Design review of the part built by this model. Coordinates are the model's own, in mm. Face numbers are marked on the shaded views. A direction names the side the tool comes from. Round coordinates to 2 decimals unless told otherwise and drop trailing zeros. Loops run counter-clockwise (first coordinate to the right, second up) from the corner with the lowest first, then second, coordinate; pieces in that order, holes last. Notation, with made-up numbers: M -9,45.25 L 24,45.25 A13 cw 24,70.25 Z; hole C -4.75,15.25 d11. An arc over 180 degrees is marked long. Use a Markdown table: item, result.
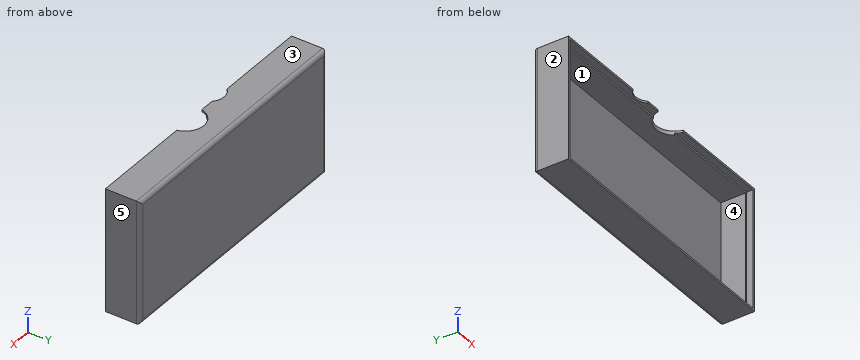
Autodesk Inventor part; units mm, degrees
sketch "Sketch8" plane through (0, 0, 0) normal (0, 1, 0) x (-1, 0, 0)
  line L0 (101.5, -46.5) -> (-101.5, -46.5)
  line L1 (-101.5, -46.5) -> (-101.5, 46.5)
  line L2 (-101.5, 46.5) -> (101.5, 46.5)
  line L3 (101.5, 46.5) -> (101.5, -46.5)
  line L4 (101.5, -46.5) -> (-101.5, 46.5) construction
  line L5 (-101.5, -46.5) -> (101.5, 46.5) construction
  point P0 (0, 0)
  dimension "d19" = 203
  dimension "d20" = 93
extrude "Extrusion4" add sketch "Sketch8" along normal blind 26.5
shell "Shell3" thickness 3 removed faces 1 at (-33.8333, 0, 15.5)
sketch "Sketch11" plane through (0, 0, 0) normal (0, 1, 0) x (-1, 0, 0)
  line L0 (-100, 45) -> (100, 45)
  line L1 (100, 45) -> (100, -45)
  line L2 (100, -45) -> (-100, -45)
  line L3 (-100, -45) -> (-100, 45)
  line L4 (-100, 45) -> (100, -45) construction
  line L5 (100, 45) -> (-100, -45) construction
  point P0 (0, 0)
  dimension "d28" = 200
  dimension "d29" = 90
extrude "Extrusion6" cut sketch "Sketch11" along normal blind 5
fillet "Fillet1" radius 3 4 edges at (0, 26.5, 46.5) (101.5, 26.5, 0) (0, 26.5, -46.5) (-101.5, 26.5, 0)
sketch "Sketch13" plane through (-101.5, 0, 46.5) normal (0, 0, 1) x (1, 0, 0)
  circle A0 centre (111.5, -3) radius 14
  circle A1 centre (78.5, -8) radius 11.5
  line L0 (-40.6, 0) -> (243.6, 0)
  line L1 (203, 0) -> (203, 23.5)
  point P0 (101.5, 0)
  dimension "d74" = 28
  dimension "d75" = 23
  dimension "d76" = 3
  dimension "d77" = 91.5
  dimension "d78" = 124.5
  dimension "d79" = 8
extrude "Extrusion8" cut sketch "Sketch13" against normal blind 10
properties part number "top"
1. Take a section at D-D on x = 4. Give the boundary of the cut face in (y, z), and give its area (3 significant figures).
Check values:
| item | result |
|---|---|
| outline | M 0,-46.5 L 23.5,-46.5 A3 ccw 26.5,-43.5 L 26.5,43.5 A3 ccw 23.5,46.5 L 9.65,46.5 L 9.65,43.5 L 23.5,43.5 L 23.5,-43.5 L 5,-43.5 L 5,-45 L 0,-45 Z |
| area | 380 mm² |
2. Take a section at B-B on x = 83.5. Give the boundary of the cut face in (y, z), and give its area (3 significant figures).
Check values:
| item | result |
|---|---|
| outline | M 0,-46.5 L 23.5,-46.5 A3 ccw 26.5,-43.5 L 26.5,43.5 A3 ccw 23.5,46.5 L 0,46.5 L 0,45 L 5,45 L 5,43.5 L 23.5,43.5 L 23.5,-43.5 L 5,-43.5 L 5,-45 L 0,-45 Z |
| area | 401 mm² |
3. Machinability: for the marked faces 1 and 2, which of the approach directions +Z, -Z, +X, -X, +Y, -Y give a long, thin tool a straight path to every point of the face, cutting with its end or side? Answer none if there is none.
Check values:
| item | result |
|---|---|
| face 1 | -Y |
| face 2 | +Z, -Z, -X, +Y, -Y |
4. Insertion check: pin 1 (1 mm diameter, centred on x = 9, y = 7, fed in from +Z); pin 2 (1 mm diameter, centred on x = -51, z = 36, fed in from -Y). Each pin has a flat end and moves straight along its axis. Give the tip position at first contact, or say it passes through.
Check values:
| item | result |
|---|---|
| pin 1 | stops at z = -43.5 |
| pin 2 | stops at y = 23.5 |
5. Wall thickness on line 1 along Z through (x, y) = (-86.5, 17.5); line 2 along X through (y, z) = (11.5, -4.5); line 3 along Z through (x, y) = (-22.5, 3.75): over which ranges is each line inside the solid? List them lowest first. Write a range as from..to.
Check values:
| item | result |
|---|---|
| line 1 | z = -46.5..-43.5, 43.5..46.5 |
| line 2 | x = -101.5..-98.5, 98.5..101.5 |
| line 3 | z = -46.5..-45, 45..46.5 |
6. The part is to be moulded in two halves that separate along X. For the marked faces 3, 4 and 5, say which applies: pulls with the +X half, pulls with the -X half, needs draft (parallel to the pull), parting line crosses it, or undercut.
Check values:
| item | result |
|---|---|
| face 3 | needs draft |
| face 4 | undercut |
| face 5 | pulls with the +X half |
7. Take a section at C-C on z = 17.5. Give the boundary of the cut face in (x, y).
Check values:
| item | result |
|---|---|
| outline | M -101.5,0 L -100,0 L -100,5 L -98.5,5 L -98.5,23.5 L 98.5,23.5 L 98.5,5 L 100,5 L 100,0 L 101.5,0 L 101.5,23.5 A3 ccw 98.5,26.5 L -98.5,26.5 A3 ccw -101.5,23.5 Z |
8. Take a section at A-A on y = 17.5. Give the boundary of the cut face in (x, z).
Check values:
| item | result |
|---|---|
| outline | M -101.5,-46.5 L 101.5,-46.5 L 101.5,46.5 L -101.5,46.5 Z; hole M -98.5,-43.5 L 98.5,-43.5 L 98.5,43.5 L -98.5,43.5 Z |
